CAD build for the part. Positions are in the model's coordinates, mm. A direction names the side the tool comes from. Give positions to 0.01 mm unless a question says otherwise; leave off trailing zeros. Loops run counter-clockwise (first coordinate to the right, second up) from the corner with the lowest first, then second, coordinate; pieces in that order, holes last.
Item 1: Saw through at A-A on x = 5. Give the cut face in (y, z), plus the area to 3 significant figures.
Item 2: Saw through at C-C on z = 34.5. Give the cut face in (x, y).
Item 3: Which spindle directions (+Z, -Z, +X, -X, +Y, -Y) get a long thin tool onto all of the face, cutting with end or side? Do faces 1 (the cylindrical face through (0.23, -82.71, -1.5)), 2 (the flat face through (5, 1, 7.071)), 3 (the flat face through (4.93, 106.017, 21.164)). Say none if no direction does.
Item 4: Drop flat-ended pins along their axis: P1, Ø5, axis at x = 8.5, y = -4, coming from the +Z side; P2, Ø1.5, axis at x = 6, y = 97.5, coming from the -Z side. Give the stop position or say it passes through.
Item 5: Probe probe 1 along Z at (x, y) = (9.5, 35); probe 2 along Y at (x, z) = (5, 36); probe 3 along Y at (x, z) = (4.25, 41). List the from-to ranges inside material, lowest first.
Item 6: Saw through at B-B on y = -34. Give the cut face in (x, z), plus the area to 3 significant figures.
from build123d import *

# Parameters (mm, degrees)
EXTRUDE_2_DEPTH = 10
SKETCH_3_R      = 5
EXTRUDE_3_DEPTH = 10


with BuildPart() as part:
    # 草图1 → 凸台-拉伸2 (new body)
    with BuildSketch(Plane(origin=(0, 0, 0), x_dir=(0, 0, -1), z_dir=(1, 0, 0))):
        with BuildLine():
            Line((-7.071067812, 77.781745931), (-7.071067812, -77.781745931))
            Line((-7.071067812, -77.781745931), (7.071067812, -77.781745931))
            Line((7.071067812, -77.781745931), (7.071067812, 77.781745931))
            ThreePointArc((7.071067812, 77.781745931), (5, 82.781745931), (0, 84.852813742))
            Line((0, 84.852813742), (-42.928932188, 127.781745931))
            ThreePointArc((-42.928932188, 127.781745931), (-55, 132.781745931), (-50, 120.710678119))
            Line((-50, 120.710678119), (-7.071067812, 77.781745931))
        make_face()
    extrude(amount=EXTRUDE_2_DEPTH)

    # 草图3 → 凸台-拉伸3 (add)
    with BuildSketch(Plane.XZ.offset(77.781745931)):
        with Locations(Location((5, 0, 0), (0, 0, 180))):
            Circle(SKETCH_3_R)
    extrude(amount=EXTRUDE_3_DEPTH)


solid = part.part
Results below:
1. outline: (-87.78, -5) - (-77.78, -5) - (-77.78, -7.07) - (77.78, -7.07) arc R7.07 ccw to (84.85, 0) - (127.78, 42.93) arc R7.07 ccw (long way) to (120.71, 50) - (77.78, 7.07) - (-77.78, 7.07) - (-77.78, 5) - (-87.78, 5) - close
1. area: 3,110 mm2
2. outline: (0, 105.21) - (10, 105.21) - (10, 119.35) - (0, 119.35) - close
3. face 1: -Y
3. face 2: +Z, +X, -X, -Y
3. face 3: -Z, +X, -X, +Y
4. P1: stops at z = 7.07
4. P2: stops at z = 11.9
5. probe 1: z = -7.07 to 7.07
5. probe 2: y = 106.71 to 120.85
5. probe 3: y = 111.71 to 125.85
6. outline: (0, -7.07) - (10, -7.07) - (10, 7.07) - (0, 7.07) - close
6. area: 141 mm2
